from build123d import *

# Parameters (mm, degrees)
SKETCH_1_R             = 3.9
EXTRUDE_1_DEPTH        = 21
HOLE_WIZARD_M4_1_D     = 3.3
HOLE_WIZARD_M5_1_D     = 4.2
HOLE_WIZARD_M5_1_DEPTH = 12
HOLE_WIZARD_M5_1_TIP   = 1.2618073
CHAMFER_1_SIZE         = 0.5


with BuildPart() as part:
    # 草图1 → 凸台-拉伸1 (new body)
    with BuildSketch(Plane(origin=(0, 0, 0), x_dir=(1, 0, 0), z_dir=(0, 1, 0))):
        Circle(SKETCH_1_R)
    extrude(amount=EXTRUDE_1_DEPTH)

    # M4 螺纹孔1 (through all)
    with Locations(Plane.XY.offset(3.9)):
        with Locations((0, 4)):
            Hole(HOLE_WIZARD_M4_1_D / 2)

    # M5 螺纹孔1
    with Locations(Plane(origin=(0, 21, 0), x_dir=(1, 0, 0), z_dir=(0, 1, 0))):
        with Locations((0, 0)):
            Hole(HOLE_WIZARD_M5_1_D / 2, depth=HOLE_WIZARD_M5_1_DEPTH)
            with Locations((0, 0, -(HOLE_WIZARD_M5_1_DEPTH + HOLE_WIZARD_M5_1_TIP / 2))):  # 118° drill point
                Cone(0, HOLE_WIZARD_M5_1_D / 2, HOLE_WIZARD_M5_1_TIP, mode=Mode.SUBTRACT)

    # 倒角1
    chamfer_1_edges = [part.edges().sort_by_distance(p)[0] for p in [
        (-3.9, 0, 0),
        (-3.9, 21, 0),
    ]]
    chamfer(chamfer_1_edges, length=CHAMFER_1_SIZE)


solid = part.part
Here's how the part is built. I have some questions about the finished solid (model axes, mm). Give positions to 0.01 mm unless a question says otherwise; leave off trailing zeros. Loops run counter-clockwise (first coordinate to the right, second up) from the corner with the lowest first, then second, coordinate; pieces in that order, holes last. Notation, with made-up numbers: (38.5, 78) -> (62.5, 78) arc R11 cw to (62.5, 95) -> close; hole circle Ø7 at (-31.5, -40). An arc over 180 degrees is marked (long way). One line per item, written item: value.
Q1. We'd pull the mould along X, two halves only. Please class faces 1 (the face through (3.72, 10.36, -1.17)), 2 (the face through (0.4, 2.4, -0.1)), 3 (the face through (0, 0, 0)), 4 (the face through (-2.003, 14.916, -0.631)): pulls with the +X half, pulls with the -X half, needs draft (parallel to the pull), parting line crosses it, or undercut.
Answers follow:
face 1: parting line crosses it
face 2: undercut
face 3: needs draft
face 4: undercut
Q2. If I drill on line 1 along Z through (x, y) = (0, 16.75); line 2 along Z through (x, y) = (1.5, 11.75); line 3 along X through (y, z) = (19.5, -1), over which ranges is the centre line in solid material (lowest first)?
Answers follow:
line 1: -3.9 to -2.1, 2.1 to 3.9
line 2: -3.6 to -1.47, 1.47 to 3.6
line 3: -3.77 to -1.85, 1.85 to 3.77
Q3. I'm going to push flat-ended pins straight in: pin 1 Ø4 at (y, z) = (3, 2.5) entering from -X; pin 2 Ø3 at (x, y) = (0, 4) entering from +Z; pin 3 Ø1.5 at (x, y) = (-2.5, 11.5) entering from -Z. Where does each tip first touch, or does it pass through?
Answers follow:
pin 1: x = -3.87
pin 2: through
pin 3: z = -3.49
Q4. Suppose I cut it at B-B on y = 4. Please give me the cut outline in (x, z).
Answers follow:
outline: (-1.65, -3.53) -> (-1.65, 3.53) arc R3.9 ccw to start; (1.65, -3.53) arc R3.9 ccw to (1.65, 3.53) -> close
Q5. Suppose I cut it at A-A on y = 16.75. Please give me the cut outline in (x, z), then the cut area to 3 significant figures.
Answers follow:
outline: circle Ø7.8 at (0, 0); hole circle Ø4.2 at (0, 0)
area: 33.9 mm^2
